```python
from build123d import *

# Parameters (mm, degrees)
BASE_FLANGE1_DEPTH           = 660.4
EDGE_FLANGE1_STRIP_W         = 14.7
EDGE_FLANGE1_STRIP_H         = 3.175
EDGE_FLANGE1_STRIP_CUT_DEPTH = 201.2
EDGE_FLANGE1_DEPTH           = 201.2


# Sheet-metal steps are written as plain solids
with BuildPart() as part:
    # Sketch1 → Base-Flange1 (new body)
    with BuildSketch(Plane.XY):
        with BuildLine():
            Line((-34.837852286, 228.6), (-34.837852286, 1))
            ThreePointArc((-34.837852286, 1), (-34.544959068, 0.292893219), (-33.837852286, 0))
            Line((-33.837852286, 0), (167.362147714, 0))
            ThreePointArc((167.362147714, 0), (168.069254495, 0.292893219), (168.362147714, 1))
            Line((168.362147714, 1), (168.362147714, 228.6))
            Line((168.362147714, 228.6), (171.537147714, 228.6))
            Line((171.537147714, 228.6), (171.537147714, 1))
            ThreePointArc((171.537147714, 1), (170.314318525, -1.952170811), (167.362147714, -3.175))
            Line((167.362147714, -3.175), (-33.837852286, -3.175))
            ThreePointArc((-33.837852286, -3.175), (-36.790023098, -1.952170811), (-38.012852286, 1))
            Line((-38.012852286, 1), (-38.012852286, 228.6))
            Line((-38.012852286, 228.6), (-34.837852286, 228.6))
        make_face()
    extrude(amount=BASE_FLANGE1_DEPTH)

    # Edge-Flange1 strip (across the edge) → Edge-Flange1 strip cut (cut)
    with BuildSketch(Plane(origin=(-33.837852286, 0, 660.4), x_dir=(0, 0, -1), z_dir=(1, 0, 0))):
        with Locations((-6.35, -1.5875)):
            Rectangle(EDGE_FLANGE1_STRIP_W, EDGE_FLANGE1_STRIP_H)
    extrude(amount=EDGE_FLANGE1_STRIP_CUT_DEPTH, mode=Mode.SUBTRACT)

    # Edge-Flange1 section (across the edge) → Edge-Flange1 (add)
    with BuildSketch(Plane(origin=(-33.837852286, 0, 660.4), x_dir=(0, 0, -1), z_dir=(1, 0, 0))):
        with BuildLine():
            Line((-3.175, 1), (-3.175, 228.6))
            Line((-3.175, 228.6), (0, 228.6))
            Line((0, 228.6), (0, 1))
            ThreePointArc((0, 1), (0.292893219, 0.292893219), (1, 0))
            Line((1, 0), (1, -3.175))
            ThreePointArc((1, -3.175), (-1.952170811, -1.952170811), (-3.175, 1))
        make_face()
    extrude(amount=EDGE_FLANGE1_DEPTH)


solid = part.part
```
Input: part model. Units: mm. Frame: model coordinates. A direction names the side the tool comes from. Coordinates: 2 decimals unless noted, no trailing zeros. Loops run counter-clockwise (first coordinate to the right, second up) from the corner with the lowest first, then second, coordinate; pieces in that order, holes last. Notation, with made-up numbers: M 14.5,-22 L 67.5,-22 A22 cw 67.5,7 Z; hole C 24.5,-20.5 d6. An arc over 180 degrees is marked long. One line per item, written item: value.
(1) Section A-A (y = 152). Output: boundary loops of the cut face in (x, z) (3 decimals), and give its area (3 significant figures).
Filled in:
outline: M -38.013,0 L -34.838,0 L -34.838,660.4 L -38.013,660.4 Z; M -33.838,660.4 L 167.362,660.4 L 167.362,663.575 L -33.838,663.575 Z; M 168.362,0 L 171.537,0 L 171.537,660.4 L 168.362,660.4 Z
area: 4,830 mm^2
(2) Line query: line 1 along X through (y, z) = (11, 368); line 2 along Y through (x, z) = (147, 373) (3 decimals); line 3 along Z through (x, y) = (130.5, 201.5) (3 decimals). Output: solid intervals per line, ascending. Write a range as from..to.
Filled in:
line 1: -38.01..-34.84, 168.36..171.54
line 2: -3.175..0
line 3: 660.4..663.575
(3) Pin query (flat end, axial travel): pin 1 (1 mm diameter, centred on x = -7.5, z = 144, fed in from +Y); pin 2 (1.3 mm diameter, centred on y = 138.5, z = 661.5, fed in from +X); pin 3 (3.5 mm diameter, centred on x = 170, y = 145.5, fed in from +Z). Return the tip coordinate at first contact, or that it passes through.
Filled in:
pin 1: y = 0
pin 2: x = 167.36
pin 3: z = 660.4
(4) Section B-B (x = -10). Output: boundary loops of the cut face in (y, z) (3 decimals), and give its area (3 significant figures).
Filled in:
outline: M -3.175,0 L 0,0 L 0,659.4 A1 cw 1,660.4 L 228.6,660.4 L 228.6,663.575 L 1,663.575 A4.175 ccw -3.175,659.4 Z
area: 2,830 mm^2
(5) Pull-direction query (X, two-part tool) for faces 4 (the flat face through (65, 116, 660.4)), 5 (the flat face through (168.362, 113, 326)), 6 (the flat face through (65, 113, 663.575)), 7 (the flat face through (171.537, 116, 326)); classes: +X half, -X half, draft (parallel to the pull), parting line (faces both ways), or undercut.
Filled in:
face 4: undercut
face 5: undercut
face 6: draft
face 7: +X half
(6) Reachability of faces 1 (the flat face through (-38.013, 113, 326)), 2 (the flat face through (-34.838, 116, 326)), 3 (the flat face through (65, 0, 325)) from +Z, -Z, +X, -X, +Y, -Y: full face, straight path, thin tool, end or side. Return the list, or none.
Filled in:
face 1: +Z, -Z, -X, +Y, -Y
face 2: +Z, -Z, +Y
face 3: -Z, +Y
(7) Section C-C (z = 363). Output: boundary loops of the cut face in (x, y) (3 decimals).
Filled in:
outline: M -38.013,1 A4.175 ccw -33.838,-3.175 L 167.362,-3.175 A4.175 ccw 171.537,1 L 171.537,228.6 L 168.362,228.6 L 168.362,1 A1 cw 167.362,0 L -33.838,0 A1 cw -34.838,1 L -34.838,228.6 L -38.013,228.6 Z
